Read the model definition and answer for the solid it produces. Units are mm, in the model's axes. Face numbers are marked on the shaded views. A direction names the side the tool comes from. Give positions to 0.01 mm unless a question says otherwise; leave off trailing zeros. Order: outer loops, then holes, each group sorted by start corner. A loop starts at its lowest first (then second) coordinate and runs counter-clockwise, first axis right, second up. Notation, with made-up numbers: M -2.5,-8 L 2.5,-8 A20 cw 2.5,7 Z; hole C 64.5,25 d2. An arc over 180 degrees is marked long. One line per item, written item: value.
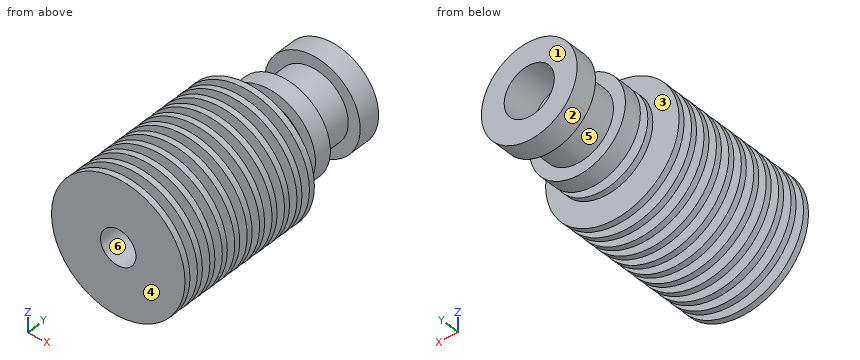
Autodesk Inventor part; units mm, degrees
ref_plane "YZ Plane" through (0, 0, 0) normal (1, 0, 0) x (0, 1, 0)
ref_plane "XZ Plane" through (0, 0, 0) normal (0, 1, 0) x (-1, 0, 0)
ref_plane "XY Plane" through (0, 0, 0) normal (0, 0, 1) x (1, 0, 0)
sketch "草圖1" plane through (0, 0, 0) normal (0, 0, 1) x (1, 0, 0)
  line L0 (0, 0) -> (-11.15, 0)
  line L1 (-11.15, 0) -> (-11.15, 1)
  line L2 (-11.15, 1) -> (0, 1)
  line L3 (0, 1) -> (0, 0)
  line L4 (0, 2.5) -> (-11.15, 2.5)
  line L5 (-11.15, 2.5) -> (-11.15, 3.5)
  line L6 (-11.15, 3.5) -> (0, 3.5)
  line L7 (0, 3.5) -> (0, 2.5)
  line L8 (0, 5) -> (-11.15, 5)
  line L9 (-11.15, 5) -> (-11.15, 6)
  line L10 (-11.15, 6) -> (0, 6)
  line L11 (0, 6) -> (0, 5)
  line L12 (0, 7.5) -> (-11.15, 7.5)
  line L13 (-11.15, 7.5) -> (-11.15, 8.5)
  line L14 (-11.15, 8.5) -> (0, 8.5)
  line L15 (0, 8.5) -> (0, 7.5)
  line L16 (0, 10) -> (-11.15, 10)
  line L17 (-11.15, 10) -> (-11.15, 11)
  line L18 (-11.15, 11) -> (0, 11)
  line L19 (0, 11) -> (0, 10)
  line L20 (0, 12.5) -> (-11.15, 12.5)
  line L21 (-11.15, 12.5) -> (-11.15, 13.5)
  line L22 (-11.15, 13.5) -> (0, 13.5)
  line L23 (0, 13.5) -> (0, 12.5)
  line L24 (0, 15) -> (-11.15, 15)
  line L25 (-11.15, 15) -> (-11.15, 16)
  line L26 (-11.15, 16) -> (0, 16)
  line L27 (0, 16) -> (0, 15)
  line L28 (0, 17.5) -> (-11.15, 17.5)
  line L29 (-11.15, 17.5) -> (-11.15, 18.5)
  line L30 (-11.15, 18.5) -> (0, 18.5)
  line L31 (0, 18.5) -> (0, 17.5)
  line L32 (0, 20) -> (-11.15, 20)
  line L33 (-11.15, 20) -> (-11.15, 21)
  line L34 (-11.15, 21) -> (0, 21)
  line L35 (0, 21) -> (0, 20)
  line L36 (0, 22.5) -> (-11.15, 22.5)
  line L37 (-11.15, 22.5) -> (-11.15, 23.5)
  line L38 (-11.15, 23.5) -> (0, 23.5)
  line L39 (0, 23.5) -> (0, 22.5)
  line L40 (0, 25) -> (-11.15, 25)
  line L41 (-11.15, 25) -> (-11.15, 26)
  line L42 (-11.15, 26) -> (0, 26)
  line L43 (0, 26) -> (0, 25)
  line L44 (-5.65, 0) -> (-4.5, 26)
  line L45 (-4.5, 26) -> (0, 26)
  line L46 (0, 0) -> (-5.65, 0)
  line L47 (0, 26) -> (0, 0)
  line L48 (0, 42.7) -> (-8, 42.7)
  line L49 (-8, 42.7) -> (-8, 39)
  line L50 (-8, 39) -> (0, 39)
  line L51 (0, 39) -> (0, 42.7)
  line L52 (-8, 33) -> (0, 33)
  line L53 (0, 33) -> (0, 30)
  line L54 (0, 30) -> (-8, 30)
  line L55 (-8, 30) -> (-8, 33)
  line L56 (-6, 39) -> (0, 39)
  line L57 (0, 39) -> (0, 33)
  line L58 (0, 33) -> (-6, 33)
  line L59 (-6, 33) -> (-6, 39)
  line L60 (-8, 28.5) -> (0, 28.5)
  line L61 (0, 28.5) -> (0, 27.5)
  line L62 (0, 27.5) -> (-8, 27.5)
  line L63 (-8, 27.5) -> (-8, 28.5)
  line L64 (-4.5, 26) -> (0, 26)
  line L65 (0, 26) -> (0, 30)
  line L66 (0, 30) -> (-4.5, 30)
  line L67 (-4.5, 30) -> (-4.5, 26)
  dimension "d2" = 11.15
  dimension "d3" = 1
  dimension "d9" = 2.5
  dimension "d11" = 5.5
  dimension "d12" = 4.5
  dimension "d14" = 42.7
  dimension "d15" = 3.7
  dimension "d16" = 3
  dimension "d17" = 8
  dimension "d19" = 6
  dimension "d20" = 6
  dimension "d21" = 1
  dimension "d22" = 1.5
revolve "迴轉1" add sketch "草圖1" angle 360 about axis through (0, 26, 0) along (0, -1, 0)
sketch "草圖2" plane through (0, 0, 0) normal (0, -1, 0) x (1, 0, 0)
  circle A0 centre (0, 0) radius 11.15
hole "孔1" at (0, 0, 0) direction (0, 1, 0) diameter 5.917 depth 14.8 tip angle 118
sketch "草圖3" plane through (0, 42.7, 0) normal (0, 1, 0) x (1, 0, 0)
  circle A0 centre (0, 0) radius 8
hole "孔2" at (0, 42.7, 0) direction (0, -1, 0) diameter 2 end through all
sketch "草圖4" plane through (0, 42.7, 0) normal (0, 1, 0) x (1, 0, 0)
  circle A0 centre (0, 0) radius 8
hole "孔3" at (0, 42.7, 0) direction (0, -1, 0) diameter 8.376 depth 6 tip angle 118
properties part number "e3d_v6_heatsink"
1) Find section D-D, the plane y = 4. Write down the section's boundary in (x, z).
Reported:
outline: C 0,0 d10.95; hole C 0,0 d5.92
2) Determine the mould class of the marked faces 4, 5 and 6 for opening direction X: +X half, -X half, draft (parallel to the pull), parting line (faces both ways), or undercut.
Reported:
face 4: draft
face 5: parting line
face 6: undercut
3) Consider probe 1 along Z at (x, y) = (0, 39.1); probe 2 along Z at (x, y) = (0, 10.75). Determine where each line is inside the solid, lowest interval first.
Reported:
probe 1: z = -8 to -4.19, 4.19 to 8
probe 2: z = -11.15 to -2.96, 2.96 to 11.15
4) Each of these flat-tipped pins is pushed along its axis until it touches: pin 1 Ø1 at (x, y) = (4.5, 36) entering from -Z; pin 2 Ø3 at (x, z) = (0, 0) entering from -Y; pin 3 Ø8 at (y, z) = (15.5, 9) entering from +X. Where does it stop, or does it pass through?
Reported:
pin 1: stops at z = -4.47
pin 2: stops at y = 15.68
pin 3: stops at x = 9.97
5) Which of the six approach directions +Z, -Z, +X, -X, +Y, -Y give full straight-line access (tool end or side, diameter ignored) to the marked faces 1, 2 and 3?
Reported:
face 1: +Z, -Z, +X, -X, +Y
face 2: +Y
face 3: none
6) Find section B-B, the plane x = 9.75. Count the separate pieces of the cut face and the enclosed holes in it, plus the area to 3 significant figures.
Reported:
separate pieces: 11
enclosed holes: 0
area: 119 mm^2
7) Find section A-A, the plane y = 25.5. Write down the section's boundary in (x, z), plus the area to 3 significant figures.
Reported:
outline: C 0,0 d22.3; hole C 0,0 d2
area: 387 mm^2
